from build123d import *

# Parameters (mm, degrees)
EXTRUDE_1_DEPTH             = 40
SKETCH_8_R                  = 1.5
CUT_EXTRUDE_2_DEPTH         = 96.336247042
SKETCH_12_W                 = 30
SKETCH_12_H                 = 40
SKETCH_12_R                 = 1.5
EXTRUDE_7_DEPTH             = 66.5
EXTRUDE_7_DIRECTION_2_REACH = 97.336
CUT_EXTRUDE_3_DEPTH         = 112.45514793
CUT_EXTRUDE_START           = -50
SKETCH_15_R                 = 3.5
CUT_EXTRUDE_4_DEPTH         = 84.791815893
SKETCH_16_W                 = 6
SKETCH_16_H                 = 21
EXTRUDE_9_DEPTH             = 10
EXTRUDE_9_DIRECTION_2_REACH = 113.455
SKETCH_17_R                 = 2
CUT_EXTRUDE_5_DEPTH         = 116.422051619


with BuildPart() as part:
    # 草图1 → 凸台-拉伸1 (new body)
    with BuildSketch(Plane(origin=(0, 0, 0), x_dir=(1, 0, 0), z_dir=(0, 1, 0))):
        Polygon((0, 0), (80, 0), (80, 6), (20, 6), (20, 27), (80, 27), (80, 33), (0, 33), align=None)
    extrude(amount=EXTRUDE_1_DEPTH)

    # 草图8 → 切除-拉伸2 (cut, through all)
    with BuildSketch(Plane(origin=(0, 0, -33), x_dir=(-1, 0, 0), z_dir=(0, 0, -1))):
        with Locations((-74, 8)):
            Circle(SKETCH_8_R)
        with Locations((-74, 32)):
            Circle(SKETCH_8_R)
        with Locations((-6, 32)):
            Circle(SKETCH_8_R)
        with Locations((-6, 8)):
            Circle(SKETCH_8_R)
    extrude(amount=-CUT_EXTRUDE_2_DEPTH, mode=Mode.SUBTRACT)

    # 草图12 → 凸台-拉伸7 (add)
    with BuildSketch(Plane.XY):
        with Locations((-5, 20)):
            Rectangle(SKETCH_12_W, SKETCH_12_H)
        with Locations((-11, 32)):
            Circle(SKETCH_12_R, mode=Mode.SUBTRACT)
        with Locations((-11, 8)):
            Circle(SKETCH_12_R, mode=Mode.SUBTRACT)
        with Locations(Location((6, 8, 0), (0, 0, 180))):
            Circle(SKETCH_12_R, mode=Mode.SUBTRACT)
        with Locations(Location((6, 32, 0), (0, 0, 180))):
            Circle(SKETCH_12_R, mode=Mode.SUBTRACT)
    extrude(amount=EXTRUDE_7_DEPTH)

    # 凸台-拉伸7 direction 2: up to this face of the body (flat: up to its plane)
    extrude_7_direction_2_end = Plane(part.part.faces().sort_by_distance((40, 20, -33))[0])
    # 草图12 → 凸台-拉伸7 direction 2 (add, up to the picked face)
    with BuildSketch(Plane.XY, mode=Mode.PRIVATE) as extrude_7_direction_2_sk1:
        with Locations((-5, 20)):
            Rectangle(SKETCH_12_W, SKETCH_12_H)
        with Locations((-11, 32)):
            Circle(SKETCH_12_R, mode=Mode.SUBTRACT)
        with Locations((-11, 8)):
            Circle(SKETCH_12_R, mode=Mode.SUBTRACT)
        with Locations(Location((6, 8, 0), (0, 0, 180))):
            Circle(SKETCH_12_R, mode=Mode.SUBTRACT)
        with Locations(Location((6, 32, 0), (0, 0, 180))):
            Circle(SKETCH_12_R, mode=Mode.SUBTRACT)
    extrude_7_direction_2_tool1 = split(extrude(extrude_7_direction_2_sk1.sketch, amount=-EXTRUDE_7_DIRECTION_2_REACH, mode=Mode.PRIVATE), bisect_by=extrude_7_direction_2_end, keep=Keep.BOTH, mode=Mode.PRIVATE)
    add(extrude_7_direction_2_tool1.solids().sort_by(Axis((-5.060326, 20, 0), (0, 0, -1)))[0])

    # 草图14 → 切除-拉伸3 (cut, through all)
    with BuildSketch(Plane(origin=(0, 40, 0), x_dir=(1, 0, 0), z_dir=(0, 1, 0))):
        Polygon((-20, 33), (0, 33), (-20, 13), align=None)
    extrude(amount=-CUT_EXTRUDE_3_DEPTH, mode=Mode.SUBTRACT)

    # 草图15 → 切除-拉伸4 (cut, through all)
    with BuildSketch(Plane.XY.offset(66.5).offset(CUT_EXTRUDE_START)):
        with Locations((-11, 32)):
            Circle(SKETCH_15_R)
        with Locations((-11, 8)):
            Circle(SKETCH_15_R)
    extrude(amount=-CUT_EXTRUDE_4_DEPTH, mode=Mode.SUBTRACT)

    # 草图16 → 凸台-拉伸9 (add)
    with BuildSketch(Plane(origin=(0, 40, 0), x_dir=(1, 0, 0), z_dir=(0, 1, 0))):
        with Locations((65, 16.5)):
            Rectangle(SKETCH_16_W, SKETCH_16_H)
    extrude(amount=EXTRUDE_9_DEPTH)

    # 凸台-拉伸9 direction 2: up to this face of the body (flat: up to its plane)
    extrude_9_direction_2_end = Plane(part.part.faces().sort_by_distance((7.48152977, 0, 9.893198609))[0])
    # 草图16 → 凸台-拉伸9 direction 2 (add, up to the picked face)
    with BuildSketch(Plane(origin=(0, 40, 0), x_dir=(1, 0, 0), z_dir=(0, 1, 0)), mode=Mode.PRIVATE) as extrude_9_direction_2_sk1:
        with Locations((65, 16.5)):
            Rectangle(SKETCH_16_W, SKETCH_16_H)
    extrude_9_direction_2_tool1 = split(extrude(extrude_9_direction_2_sk1.sketch, amount=-EXTRUDE_9_DIRECTION_2_REACH, mode=Mode.PRIVATE), bisect_by=extrude_9_direction_2_end, keep=Keep.BOTH, mode=Mode.PRIVATE)
    add(extrude_9_direction_2_tool1.solids().sort_by(Axis((65, 40, -16.5), (0, -1, 0)))[0])

    # 草图17 → 切除-拉伸5 (cut, through all)
    with BuildSketch(Plane.XY):
        with Locations((32, 25)):
            Circle(SKETCH_17_R)
    extrude(amount=-CUT_EXTRUDE_5_DEPTH, mode=Mode.SUBTRACT)


solid = part.part
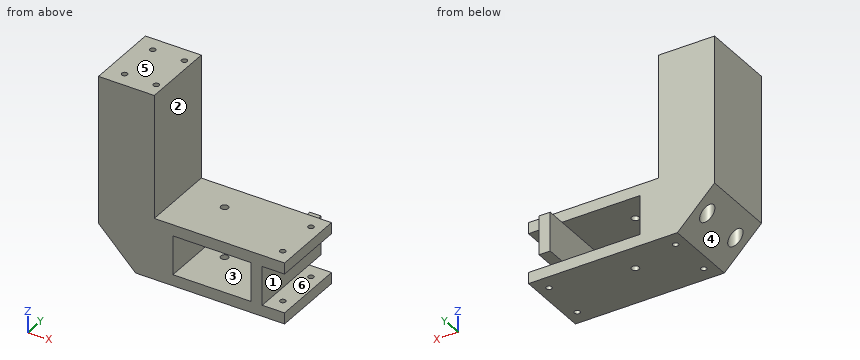
Build history of the part. All positions in model axes, mm. Face numbers are marked on the shaded views. A direction names the side the tool comes from. Coordinates: 2 decimals unless noted, no trailing zeros. Write each loop counter-clockwise with the first axis right and the second up, starting at its lowest first coordinate (ties: lowest second). Pieces come first, ordered by that corner, then holes.
(1) 3-axis set-ups, long thin cutter, end or side, ignore diameter. For the marked faces 1, 2 and 3: which of +Z, -Z, +X, -X, +Y, -Y reach the whole face in a straight line?
(2) Cut at D-D on x = -11. List the corners of the cut face in (y, z).
(3) Pin check, flat tips, straight feed: pin 1 Ø10.5 at (y, z) = (18.5, -21.5) entering from +X; pin 2 Ø10 at (y, z) = (28.5, 30) entering from +X; pin 3 Ø3.5 at (x, y) = (74, 8) entering from +Z; pin 4 Ø3.5 at (x, y) = (32, 25) entering from +Z. Stop position of each tip, or through.
(4) Cut at C-C on y = 15. List the corners of the cut face in (x, z), and give its area (3 significant figures).
(5) Drill centre lines: line 1 (X direction, y = 32, z = 8); line 2 (Y direction, x = 74, z = -30.6); line 3 (Z direction, x = 27, y = 28.5). Where is each one in solid material? Low to high.
(6) Cut at A-A on z = -3. List the corners of the cut face in (x, y), and give its area (3 significant figures).
(7) Mould opens along Z. For the marked faces 4, 5 and 6 say: pulls with the +Z half, pulls with the -Z half, needs draft (parallel to the pull), parting line crosses it, or undercut.
(8) Cut at B-B on x = 32. List the corners of the cut face in (y, z).
Working result:
1. face 1: +X, +Y, -Y
1. face 2: +Z, +X, +Y, -Y
1. face 3: +Y, -Y
2. outline: (0, -22) - (4.5, -22) - (4.5, 16.5) - (6.5, 16.5) - (6.5, 66.5) - (0, 66.5) - close; (9.5, 16.5) - (11.5, 16.5) - (11.5, -22) - (28.5, -22) - (28.5, 16.5) - (30.5, 16.5) - (30.5, 66.5) - (9.5, 66.5) - close; (33.5, 16.5) - (35.5, 16.5) - (35.5, -22) - (40, -22) - (40, 66.5) - (33.5, 66.5) - close
3. pin 1: stops at x = 68
3. pin 2: stops at x = 10
3. pin 3: stops at z = 0
3. pin 4: passes through
4. outline: (-20, -13) - (0, -33) - (80, -33) - (80, -27) - (68, -27) - (68, -6) - (80, -6) - (80, 0) - (10, 0) - (10, 66.5) - (-20, 66.5) - close; hole (20, -27) - (62, -27) - (62, -6) - (20, -6) - close
4. area: 3,960 mm2
5. line 1: x = -20 to -14.5, -7.5 to 4.5, 7.5 to 10
5. line 2: y = 0 to 6.5, 9.5 to 30.5, 33.5 to 40
5. line 3: z = -33 to -27, -6 to 0
6. outline: (-20, 0) - (80, 0) - (80, 40) - (-20, 40) - close; hole circle Ø7 at (-11, 8); hole circle Ø7 at (-11, 32); hole circle Ø3 at (6, 8); hole circle Ø3 at (6, 32); hole circle Ø4 at (32, 25); hole circle Ø3 at (74, 8); hole circle Ø3 at (74, 32)
6. area: 3,880 mm2
7. face 4: pulls with the -Z half
7. face 5: pulls with the +Z half
7. face 6: undercut
8. outline: (0, -33) - (23, -33) - (23, -27) - (0, -27) - close; (0, -6) - (23, -6) - (23, 0) - (0, 0) - close; (27, -33) - (40, -33) - (40, -27) - (27, -27) - close; (27, -6) - (40, -6) - (40, 0) - (27, 0) - close
